Model file for the job. Use its own axes, mm. A direction names the side the tool comes from. Give positions to 0.01 mm unless a question says otherwise; leave off trailing zeros. Loops run counter-clockwise (first coordinate to the right, second up) from the corner with the lowest first, then second, coordinate; pieces in that order, holes last. Notation, with made-up numbers: M 13,52.5 L 33,52.5 A12 ccw 33,60.5 Z; hole C 48,52.25 d8. An arc over 180 degrees is marked long. Use CSV: the item, a comma, the result in double quotes. Start each with the question number.
(1) Tool access for faces 4 (the face through (78, 146.667, 26)), 5 (the face through (78, 121.667, 48)), 6 (the face through (78.4, 141.066, 43.197)), 7 (the face through (78, 119, 5)): list every direction of +Z, -Z, +X, -X, +Y, -Y with a clear straight run to the whole face (end or side of a thin tool).
(2) Wall check: line 1 along Y through (x, z) = (67.5, 36); line 2 along Z through (x, y) = (83, 105); line 3 along Z through (x, y) = (77, 124). Give the ranges that are in metal, low to high. Write a range as from..to.
(3) Slice it at A-A on x = 70.25. List the corners of the cut face in (y, z).
(4) Slice it at C-C on z = 6. List the corners of the cut face in (x, y) (3 decimals).
(5) Flat gauge pins, fed straight in: P1, Ø1, axis at x = 74.5, z = 22, coming from the -Y side; P2, Ø4, axis at x = 78, y = 102, coming from the +Z side; P3, Ø6.5, axis at x = 81.5, y = 114, coming from the -Z side. Where does each tip first touch, or does it go through?
(6) Slice it at D-D on x = 81.5. List the corners of the cut face in (y, z), and give its area (3 significant figures).
(7) Slice it at B-B on y = 118. List the corners of the cut face in (x, z) (3 decimals).
(8) Two-plate mould, pull along X, no slides. Class faces 1 (the face through (78, 141.667, 22)), 2 (the face through (78, 122, 0.95)), 3 (the face through (91.075, 142, 21)): pulls with the +X half, pulls with the -X half, needs draft (parallel to the pull), parting line crosses it, or undercut.
Autodesk Inventor part; units mm, degrees
ref_plane "XZ Plane" through (0, 0, 0) normal (0, 1, 0) x (-1, 0, 0)
ref_plane "XY Plane" through (0, 0, 0) normal (0, 0, 1) x (1, 0, 0)
ref_plane "Work Plane1" through (78.575, 0, 0) normal (1, 0, 0) x (0, 1, 0)
sketch "Sketch2" plane through (78.575, 0, 0) normal (1, 0, 0) x (0, 1, 0)
  line L0 (-170.29, 0) -> (141.6673, 38.3035)
  line L1 (141.6673, 38.3035) -> (140.4486, 48.229)
  line L2 (-171.5087, 9.9255) -> (140.4486, 48.229)
  line L3 (-170.29, 0) -> (-171.5087, 9.9255)
  line L4 (-304.8, 0) -> (304.8, 0)
  line L5 (-304.8, 0) -> (-304.8, -25.4)
  line L6 (304.8, -25.4) -> (-304.8, -25.4)
  line L7 (304.8, 0) -> (304.8, -25.4)
  line L8 (141.6673, 0) -> (146.6673, 0)
  line L9 (146.6673, 0) -> (146.6673, 53.4221)
  line L10 (146.6673, 53.4221) -> (141.6673, 53.4221)
  line L11 (141.6673, 53.4221) -> (141.6673, 0)
  line L12 (141.6673, 53.4221) -> (121.6673, 53.4221)
  line L13 (121.6673, 53.4221) -> (121.6673, 38.3035)
  line L14 (121.6673, 38.3035) -> (141.6673, 38.3035)
  line L15 (141.6673, 38.3035) -> (141.6673, 53.4221)
  line L16 (141.6673, 38.3035) -> (140.4486, 48.229)
  line L17 (121.6673, 45.8628) -> (140.4486, 48.229)
  line L18 (146.6673, 0) -> (96.6673, 0)
  line L19 (96.6673, 0) -> (96.6673, 5)
  line L20 (96.6673, 5) -> (146.6673, 5)
  line L21 (146.6673, 5) -> (146.6673, 0)
  line L22 (141.6673, 53.4221) -> (121.6673, 50.9023)
  line L23 (101.6673, 0) -> (141.6673, 0)
  line L24 (141.6673, 0) -> (141.6673, 0.95)
  line L25 (141.6673, 0.95) -> (101.6673, 0.95)
  line L26 (101.6673, 0.95) -> (101.6673, 0)
  point P0 (0, 0)
  point P1 (141.6673, 5)
  point P2 (121.6673, 45.9229)
  dimension "d2" = 5
  dimension "d3" = 20
  dimension "d4" = 50
  dimension "d5" = 5
  dimension "d6" = 5
  dimension "d7" = 40
  dimension "d8" = 5
  dimension "d9" = 0.95
extrude "Extrusion1" add sketch "Sketch2" along normal mid plane 25 contours L1 L2 L13 L22 L11 | L11 L10 L9 L20 | L19 L20 L11 L25 L26 L4 | L20 L9 L4 L11 | L26 L25 L11 L4
extrude "Extrusion2" cut sketch "Sketch2" along normal mid plane 13.2 contours L26 L25 L11 L4
properties part number "coverHolder_CPY"
Reply:
1,face 4,"+Z, -Z, +X, -X, +Y"
1,face 5,"+Z, +X, -X, -Y"
1,face 6,"+X, -X"
1,face 7,"+X, -X, -Y"
2,line 1,"y = 141.67..146.67"
2,line 2,"z = 0.95..5"
2,line 3,"z = 0.95..5, 46.21..51.2"
3,outline,"M 96.67,0 L 146.67,0 L 146.67,53.42 L 141.67,53.42 L 121.67,50.9 L 121.67,45.92 L 140.45,48.23 L 141.67,38.3 L 141.67,5 L 96.67,5 Z"
4,outline,"M 66.075,141.667 L 91.075,141.667 L 91.075,146.667 L 66.075,146.667 Z"
5,P1,"stops at y = 141.67"
5,P2,"stops at z = 5"
5,P3,"stops at z = 0.95"
6,outline,"M 96.67,0 L 101.67,0 L 101.67,0.95 L 141.67,0.95 L 141.67,0 L 146.67,0 L 146.67,53.42 L 141.67,53.42 L 121.67,50.9 L 121.67,45.92 L 140.45,48.23 L 141.67,38.3 L 141.67,5 L 96.67,5 Z"
6,area,"560 mm^2"
7,outline,"M 66.075,0 L 71.975,0 L 71.975,0.95 L 85.175,0.95 L 85.175,0 L 91.075,0 L 91.075,5 L 66.075,5 Z"
8,face 1,"needs draft"
8,face 2,"undercut"
8,face 3,"pulls with the +X half"
